Geometry: see drawing. Coordinates: mm, zero at the bounding-box minimum. Coordinates: 2 decimals unless noted, no trailing zeros. Loops run counter-clockwise (first coordinate to the right, second up) from the corner with the lowest first, then second, coordinate; pieces in that order, holes last. Notation, with made-up numbers: (7, 77) -> (20, 77) arc R22 ccw to (20, 90) -> close; hole circle Ø6 at (30, 43.25). An arc over 180 degrees is marked (long way). One line per item, written item: value. Start each with the question number.
Item 1: Section query C-C on z = 9.5. Return loops of the section in (x, y), then the cut area to 3 significant figures.
Item 2: Section query A-A on y = 5. Return loops of the section in (x, z), then the cut area to 3 significant figures.
Item 3: Ray query, probe 1 along Z at (x, y) = (43, 2.75); probe 2 along Y at (x, z) = (60, 7.5); probe 3 along X at (y, z) = (5.25, 9.5). Return the intervals inside material, ascending. Write a range as from..to.
Item 4: Section query D-D on x = 20. Return loops of the section in (y, z).
Item 5: Section query B-B on x = 43. Return loops of the section in (y, z).
Item 6: Contact query for a flat-ended pin moving along its axis: pin 1 Ø4 at (x, y) = (60, 5) entering from -Z. Output: stop coordinate, or through.
Item 7: Mould query, pull axis X, two halves, no side actions, for the marked faces 1, 2 and 3. Classes: +X half, -X half, draft (parallel to the pull), parting line (faces both ways), or undercut.
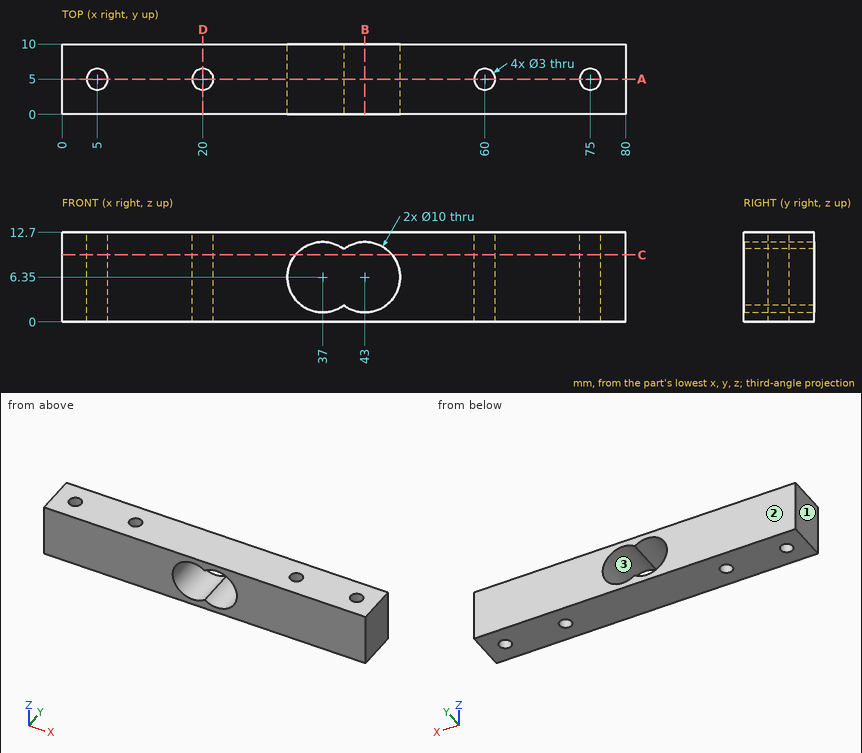
Reply:
1. outline: (0, 0) -> (33.12, 0) -> (33.12, 10) -> (0, 10) -> close; (46.88, 0) -> (80, 0) -> (80, 10) -> (46.88, 10) -> close; hole circle Ø3 at (5, 5); hole circle Ø3 at (20, 5); hole circle Ø3 at (60, 5); hole circle Ø3 at (75, 5)
1. area: 634 mm²
2. outline: (0, 0) -> (3.5, 0) -> (3.5, 12.7) -> (0, 12.7) -> close; (6.5, 0) -> (18.5, 0) -> (18.5, 12.7) -> (6.5, 12.7) -> close; (21.5, 0) -> (58.5, 0) -> (58.5, 12.7) -> (21.5, 12.7) -> close; (61.5, 0) -> (73.5, 0) -> (73.5, 12.7) -> (61.5, 12.7) -> close; (76.5, 0) -> (80, 0) -> (80, 12.7) -> (76.5, 12.7) -> close; hole (40, 2.35) arc R5 ccw (long way) to (40, 10.35) arc R5 ccw (long way) to start
2. area: 729 mm²
3. probe 1: z = 0..1.35, 11.35..12.7
3. probe 2: y = 0..3.5, 6.5..10
3. probe 3: x = 0..3.52, 6.48..18.52, 21.48..33.12, 46.88..58.52, 61.48..73.52, 76.48..80
4. outline: (0, 0) -> (3.5, 0) -> (3.5, 12.7) -> (0, 12.7) -> close; (6.5, 0) -> (10, 0) -> (10, 12.7) -> (6.5, 12.7) -> close
5. outline: (0, 0) -> (10, 0) -> (10, 1.35) -> (0, 1.35) -> close; (0, 11.35) -> (10, 11.35) -> (10, 12.7) -> (0, 12.7) -> close
6. pin 1: stops at z = 0
7. face 1: -X half
7. face 2: draft
7. face 3: undercut
